Autodesk Inventor part; units mm, degrees
ref_plane "YZ Plane" through (0, 0, 0) normal (1, 0, 0) x (0, 1, 0)
ref_plane "XZ Plane" through (0, 0, 0) normal (0, 1, 0) x (-1, 0, 0)
ref_plane "XY Plane" through (0, 0, 0) normal (0, 0, 1) x (1, 0, 0)
sketch "Skizze1" plane through (0, 0, 0) normal (0, 0, 1) x (1, 0, 0)
  line L0 (-14.4, 0) -> (2.4, 0)
  line L1 (0, -3.2) -> (0, 19.2)
  line L2 (0, 15) -> (-1, 15)
  line L3 (-1, 15) -> (-2, 14)
  line L4 (-2, 14) -> (-6, 14)
  line L5 (-6, 14) -> (-7, 15)
  line L6 (-7, 15) -> (-10, 15)
  line L7 (-10, 15) -> (-10, 13.5)
  line L8 (-0.5, 16) -> (-11.5, 16)
  line L9 (-12, 15.5) -> (-12, 12.5)
  line L10 (-12, 12.5) -> (-11, 12.5)
  line L11 (-11, 12.5) -> (-10, 13.5)
  line L12 (-11.5, 16) -> (-12, 15.5)
  line L13 (0, 15.5) -> (0, 15)
  line L14 (0, 15.5) -> (-0.5, 16)
  point P0 (0, 0)
  point P1 (0, 16)
  point P2 (-12, 16)
  dimension "d0" = 28
  dimension "d1" = 30
  dimension "d2" = 45
  dimension "d3" = 45
  dimension "d4" = 1
  dimension "d5" = 10
  dimension "d6" = 3
  dimension "d7" = 12
  dimension "d9" = 25
  dimension "d10" = 1
  dimension "d11" = 0.5
  dimension "d12" = 0.5
  dimension "d13" = 0.5
  dimension "d14" = 0.5
  dimension "d25" = 27
  dimension "d26" = 1
revolve "Umdrehung1" add sketch "Skizze1" angle 360 about axis through (-10, 0, 0) along (1, 0, 0)
hole "Bohrung1" at (0, 0, 0) direction (-1, 0, 0) diameter 28.917 depth 8
properties part number "13_0204_036"
Check sheet for the modelled part. Datum: model origin and axes. Units: mm. A direction names the side the tool comes from. Give positions to 0.01 mm unless a question says otherwise; leave off trailing zeros. Write each loop counter-clockwise with the first axis right and the second up, starting at its lowest first coordinate (ties: lowest second). Pieces come first, ordered by that corner, then holes.
Item 1: Access from +Z, -Z, +X, -X, +Y, -Y to the whole of each face (thin tool, end or side, straight path). Record for faces 1 (the face through (-4.03, -4.34, -13.79)), 2 (the face through (0, -8, 13)).
Item 2: Gauge pin test, flat ends, axial feed: pin 1 (4 mm diameter, centred on y = -5.5, z = -10.5, fed in from +X); pin 2 (6 mm diameter, centred on x = -1.5, z = -9, fed in from -Y); pin 3 (4 mm diameter, centred on x = -3.5, y = 10, fed in from -Z). Record the tip position at first contact, or that the pin passes through.
Item 3: Cross-section at C-C (x = -5.5). Enter the section's corners in (y, z).
Item 4: Draft check along Y on faces 3 (the face through (-6.08, -3.47, 15.62)), 4 (the face through (-10, -11.18, 7.85)), 5 (the face through (-8.521, -14.985, -0.66)), 6 (the face through (-12, 1, 13)). Enter one of: released by +Y, released by -Y, zero draft, split by the parting line, or undercut.
Item 5: Scan lines: L1, parallel to Z at x = -0.5, y = 0; L2, parallel to Z at x = -11.5, y = 0; L3, parallel to Y at x = -2.25, z = 7. Record each from-to range of solid material in increasing order.
Item 6: Cross-section at A-A (y = 0). Enter the section's corners in (x, z).
Report:
1. face 1: +X
1. face 2: +Z, -Z, +X, +Y, -Y
2. pin 1: stops at x = -10
2. pin 2: stops at y = -14.83
2. pin 3: stops at z = -13.86
3. outline: circle Ø32 at (0, 0); hole circle Ø28.92 at (0, 0)
4. face 3: split by the parting line
4. face 4: undercut
4. face 5: undercut
4. face 6: zero draft
5. L1: z = -16 to -15, 15 to 16
5. L2: z = -16 to -12.5, 12.5 to 16
5. L3: y = -14.39 to -12.65, 12.65 to 14.39
6. outline: (-12, -15.5) - (-11.5, -16) - (-0.5, -16) - (0, -15.5) - (0, -15) - (-1, -15) - (-1.54, -14.46) - (-6.46, -14.46) - (-7, -15) - (-10, -15) - (-10, -13.5) - (-11, -12.5) - (-12, -12.5) - close; (-12, 12.5) - (-11, 12.5) - (-10, 13.5) - (-10, 15) - (-7, 15) - (-6.46, 14.46) - (-1.54, 14.46) - (-1, 15) - (0, 15) - (0, 15.5) - (-0.5, 16) - (-11.5, 16) - (-12, 15.5) - close
